```python
from build123d import *

# Parameters (mm, degrees)
F1_DEPTH  = 6.25
F3_DEPTH  = 6.25
F5_DEPTH  = 6.25
F6_R      = 2.05
F6_R_2    = 3.05
F7_DEPTH  = 25
F8_R      = 2.05
F9_DEPTH  = 25
F10_R     = 2.05
F11_DEPTH = 25
F13_R     = 3.55
F14_DEPTH = 3
F15_R     = 3.55
F16_DEPTH = 3
F17_R     = 3.55
F17_R_2   = 4.55
F18_DEPTH = 3
F19_SIZE  = 5
F20_SIZE  = 3
F21_SIZE  = 3


with BuildPart() as f1:
    # F0 (on Top) → F1 (new body)
    with BuildSketch(Plane.XY):
        Polygon((4.1484118214, 32.5575917727), (-22.1015881786, 32.5575917727), (-22.1015881786, -13.6924082273), (24.1484118214, -13.6924082273), (24.1484118214, 12.5575917727), align=None)
    extrude(amount=F1_DEPTH)

    # F6 (on face) → F7 (cut)
    with BuildSketch(Plane.XY.offset(6.25)):
        with Locations((-5.8515881786, 22.5575917727)):
            Circle(F6_R)
        with Locations((-5.8515881786, 2.5575917727)):
            Circle(F6_R_2)
        with Locations((14.1484118214, 2.5575917727)):
            Circle(F6_R)
    extrude(amount=-F7_DEPTH, mode=Mode.SUBTRACT)


with BuildPart() as f3:
    # F2 (on face) → F3 (new body)
    with BuildSketch(Plane.XZ.offset(13.6924082273)):
        Polygon((-22.1015881786, 46.25), (-22.1015881786, 6.25), (24.1484118214, 6.25), (24.1484118214, 32.5), (4.1484118214, 46.25), align=None)
    extrude(amount=-F3_DEPTH)

    # F8 (on face) → F9 (cut)
    with BuildSketch(Plane(origin=(0, -7.4424082273, 0), x_dir=(-1, 0, 0), z_dir=(0, 1, 0))):
        with Locations((5.8515881786, 16.25)):
            Circle(F8_R)
        with Locations((-14.1484118214, 16.25)):
            Circle(F8_R)
        with Locations((5.8515881786, 36.25)):
            Circle(F8_R)
    extrude(amount=-F9_DEPTH, mode=Mode.SUBTRACT)


with BuildPart() as f5:
    # F4 (on face) → F5 (new body)
    with BuildSketch(Plane(origin=(-22.1015881786, 0, 0), x_dir=(0, -1, 0), z_dir=(-1, 0, 0))):
        Polygon((-32.5575917727, 6.25), (7.4424082273, 6.25), (7.4424082273, 46.25), (-18.8075917727, 46.25), (-32.5575917727, 32.5), align=None)
    extrude(amount=-F5_DEPTH)

    # F10 (on face) → F11 (cut)
    with BuildSketch(Plane.YZ.offset(-15.8515881786)):
        with Locations((22.5575917727, 16.25)):
            Circle(F10_R)
        with Locations((2.5575917727, 16.25)):
            Circle(F10_R)
        with Locations((2.5575917727, 36.25)):
            Circle(F10_R)
    extrude(amount=-F11_DEPTH, mode=Mode.SUBTRACT)


with BuildPart() as f1_1:
    add(f1.part)

    # F12: union F3, F5
    add(f3.part)
    add(f5.part)

    # F13 (on face) → F14 (cut)
    with BuildSketch(Plane.XZ.offset(13.6924082273)):
        with Locations((-5.8515881786, 36.25)):
            Circle(F13_R)
        with Locations((14.1484118214, 16.25)):
            Circle(F13_R)
        with Locations((-5.8515881786, 16.25)):
            Circle(F13_R)
    extrude(amount=-F14_DEPTH, mode=Mode.SUBTRACT)

    # F15 (on face) → F16 (cut)
    with BuildSketch(Plane(origin=(-22.1015881786, 0, 0), x_dir=(0, -1, 0), z_dir=(-1, 0, 0))):
        with Locations((-2.5575917727, 36.25)):
            Circle(F15_R)
        with Locations((-2.5575917727, 16.25)):
            Circle(F15_R)
        with Locations((-22.5575917727, 16.25)):
            Circle(F15_R)
    extrude(amount=-F16_DEPTH, mode=Mode.SUBTRACT)

    # F17 (on face) → F18 (cut)
    with BuildSketch(Plane(origin=(0, 0, 0), x_dir=(1, 0, 0), z_dir=(0, 0, -1))):
        with Locations((-5.8515881786, -22.5575917727)):
            Circle(F17_R)
        with Locations((-5.8515881786, -2.5575917727)):
            Circle(F17_R_2)
        with Locations((14.1484118214, -2.5575917727)):
            Circle(F17_R)
    extrude(amount=-F18_DEPTH, mode=Mode.SUBTRACT)

    # F19
    f19_edges = [f1_1.edges().sort_by_distance(p)[0] for p in [
        (-22.101588, -13.692408, 23.125),
    ]]
    chamfer(f19_edges, length=F19_SIZE)

    # F20 (call 1 of 2: OpenCascade refuses the feature's edges together)
    f20_edges = [f1_1.edges().sort_by_distance(p)[0] for p in [
        (-6.476588, -13.692408, 46.25),
        (14.148412, -13.692408, 39.375),
        (24.148412, -13.692408, 16.25),
    ]]
    chamfer(f20_edges, length=F20_SIZE)

    # F20#2 (call 2 of 2)
    f20_2_edges = [f1_1.edges().sort_by_distance(p)[0] for p in [
        (-22.101588, 5.057592, 46.25),
        (-22.101588, 25.682592, 39.375),
        (-22.101588, 32.557592, 16.25),
    ]]
    chamfer(f20_2_edges, length=F20_SIZE)

    # F21
    f21_edges = [f1_1.edges().sort_by_distance(p)[0] for p in [
        (22.648412, -12.192408, 0),
        (24.148412, 0.932592, 0),
        (14.148412, 22.557592, 0),
        (-7.476588, 32.557592, 0),
        (-20.601588, 31.057592, 0),
        (-22.101588, 10.432592, 0),
        (-19.601588, -11.192408, 0),
        (2.023412, -13.692408, 0),
    ]]
    chamfer(f21_edges, length=F21_SIZE)


solid = f1_1.part
```
Here's how the part is built. I have some questions about the finished solid (model axes, mm). A direction names the side the tool comes from. Coordinates: 2 decimals unless noted, no trailing zeros. Loops run counter-clockwise (first coordinate to the right, second up) from the corner with the lowest first, then second, coordinate; pieces in that order, holes last. Notation, with made-up numbers: (89, -18.75) - (119, -18.75) arc R31 cw to (119, 11.25) - close; hole circle Ø9 at (-30, 15). An arc over 180 degrees is marked (long way). Answer as CSV lines item,"result".
Q1. If we section it at A-A, the plane z = 37.5: Write out the boundary of the cut face in (x, y), and give its area (3 significant figures).
Response:
outline,"(-22.1, -8.69) - (-17.1, -13.69) - (-9.17, -13.69) - (-9.17, -10.69) - (-7.48, -10.69) - (-7.48, -7.44) - (-15.85, -7.44) - (-15.85, 0.93) - (-19.1, 0.93) - (-19.1, -0.77) - (-22.1, -0.77) - close; (-22.1, 5.88) - (-19.1, 5.88) - (-19.1, 4.18) - (-15.85, 4.18) - (-15.85, 27.56) - (-19.1, 27.56) - (-22.1, 23.31) - close; (-4.23, -10.69) - (-2.53, -10.69) - (-2.53, -13.69) - (11.58, -13.69) - (16.88, -10.69) - (16.88, -7.44) - (-4.23, -7.44) - close"
area,"375 mm2"
Q2. If we section it at B-B, the plane z = 30: Write out the boundary of the cut face in (x, y), and give its area (3 significant figures).
Response:
outline,"(-22.1, -8.69) - (-17.1, -13.69) - (21.15, -13.69) - (24.15, -10.69) - (24.15, -7.44) - (-15.85, -7.44) - (-15.85, 32.56) - (-19.1, 32.56) - (-22.1, 29.56) - close"
area,"518 mm2"
Q3. We'd pull the mould along Z, two halves only. Please class faces 5 (the face through (-19.102, 3, 34)), 6 (the face through (-22.102, 11, 23)), 7 (the face through (-5, 6, 3)), 8 (the face through (14.29, -9.09, 39.28)): pulls with the +Z half, pulls with the -Z half, needs draft (parallel to the pull), parting line crosses it, or undercut.
Response:
face 5,"undercut"
face 6,"needs draft"
face 7,"pulls with the -Z half"
face 8,"pulls with the +Z half"
Q4. If we section it at C-C, the plane x = 5: Write out the boundary of the cut face in (y, z).
Response:
outline,"(-13.69, 3) - (-10.69, 0) - (27.46, 0) - (31.71, 3) - (31.71, 6.25) - (-7.44, 6.25) - (-7.44, 45.66) - (-10.69, 45.66) - (-13.69, 42.02) - close"
Q5. For pin 1 (4.5 mm diameter, centred on x = -6, y = 3.5, fed in from -Z); pin 2 (6 mm diameter, centred on x = -3.5, z = 18, fed in from +Y); pin 3 (3 mm diameter, centred on x = 7.5, y = 0.5, fed in from +Z); pin 4 (3.5 mm diameter, centred on y = 22.56, z = 16.25, fed in from -X), each with a flat end and sliding along its axis, tell me the tip position at first contact or that it passes through.
Response:
pin 1,"z = 3"
pin 2,"y = -7.44"
pin 3,"z = 6.25"
pin 4,"through"
Q6. If I drill on L1, parallel to X at y = -9, z = 16; L2, parallel to X at y = 26.5, z = 16.5; L3, parallel to Y at x = -6.5, z = 28.5, over which ranges is the centre line in solid material (lowest first)? Write a range as [from, to].
Response:
L1,"[-21.79, -7.89], [-3.82, 12.11], [16.18, 24.15]"
L2,"[-22.1, -15.85]"
L3,"[-13.69, -7.44]"
Q7. For faces 1 (the face through (-20.62, 3.02, 19.77)), 2 (the face through (4, -7.442, 27)), 3 (the face through (-4, 24, 3)), 4 (the face through (16, -10.692, 15)), which set-ups out of +Z, -Z, +X, -X, +Y, -Y let a thin tool reach every point of the face, with its end or its side?
Response:
face 1,"-X"
face 2,"+Z, +X, +Y"
face 3,"-Z"
face 4,"-Y"
Q8. If we section it at D-D, the plane z = 16.25: Give the number of separate pieces and of enclosed holes in the cut face, and give its area (3 significant figures).
Response:
separate pieces,"5"
enclosed holes,"0"
area,"379 mm2"
